Check sheet for the modelled part. Datum: model origin and axes. Units: mm. A direction names the side the tool comes from. Round coordinates to 2 decimals unless told otherwise and drop trailing zeros. Order: outer loops, then holes, each group sorted by start corner. A loop starts at its lowest first (then second) coordinate and runs counter-clockwise, first axis right, second up. Notation, with made-up numbers: M 67,79 L 108,79 A31 ccw 108,112 Z; hole C 18,32.5 d5. An arc over 180 degrees is marked long. One line per item, written item: value. Start each with the question number.
(1) Cross-section at C-C, the plane z = -9.25. Enter the section's corners in (x, y), and give its area (3 significant figures).
(2) Release check for a two-part mould opening along Y. For faces 1 (the face through (4.52, 14.77, -8.5)), 2 (the face through (15.86, 11.62, -1.48)), 3 (the face through (10, 8, 0)), 4 (the face through (13, 0, -10)) record: released by +Y, released by -Y, zero draft, split by the parting line, or undercut.
(3) Access from +Z, -Z, +X, -X, +Y, -Y to the whole of each face (thin tool, end or side, straight path). Record for faces 5 (the face through (3, 12, -12)), 6 (the face through (12, 8, -3)), 7 (the face through (10, 8, -20)).
(4) Thickness scan on L1, parallel to Z at x = 5.25, y = 10; L2, parallel to Y at x = 4.05, z = -10; L3, parallel to Z at x = 12.75, y = 6. Record the ranges inside material, lowest first.
(5) Cross-section at B-B, the plane x = 16. Enter the section's corners in (y, z), and give its area (3 significant figures).
(6) Depth check by flat-ended pin: pin 1 Ø4 at (y, z) = (17, -7) entering from -X; pin 2 Ø6 at (x, z) = (21.5, -11) entering from +Y; pin 3 Ø8 at (y, z) = (9.5, -11) entering from +X. Enter the tip coordinate at first touch or a pass-through.
(7) Cross-section at A-A, the plane y = 2.5. Enter the section's corners in (x, z), and give its area (3 significant figures).
(8) Cross-section at D-D, the plane y = 10.75. Enter the section's corners in (x, z).
from build123d import *

# Parameters (mm, degrees)
SKETCH_1_W          = 40
SKETCH_1_H          = 20
EXTRUDE_1_DEPTH     = 20
SKETCH_2_W          = 34
SKETCH_2_H          = 14
CUT_EXTRUDE_1_DEPTH = 20
CUT_EXTRUDE_2_DEPTH = 20
SKETCH_5_R          = 5
CUT_EXTRUDE_3_DEPTH = 3
SKETCH_6_W          = 34
SKETCH_6_H          = 20
CUT_EXTRUDE_4_DEPTH = 3
SKETCH_7_W          = 14
SKETCH_7_H          = 20
CUT_EXTRUDE_5_DEPTH = 3
EXTRUDE_2_DEPTH     = 3
EXTRUDE_3_DEPTH     = 3


with BuildPart() as part:
    # 草图1 → 凸台-拉伸1 (new body)
    with BuildSketch(Plane(origin=(0, 0, 0), x_dir=(1, 0, 0), z_dir=(0, 1, 0))):
        with Locations((20, 10)):
            Rectangle(SKETCH_1_W, SKETCH_1_H)
    extrude(amount=EXTRUDE_1_DEPTH)

    # 草图2 → 切除-拉伸1 (cut)
    with BuildSketch(Plane.XY):
        with Locations((23, 13)):
            Rectangle(SKETCH_2_W, SKETCH_2_H)
    extrude(amount=-CUT_EXTRUDE_1_DEPTH, mode=Mode.SUBTRACT)

    # 草图4 → 切除-拉伸2 (cut)
    with BuildSketch(Plane.ZY):
        with BuildLine():
            ThreePointArc((-7.4, 10), (-9.005023076, 12.402086785), (-11.838477631, 11.838477631))
            Line((-11.838477631, 11.838477631), (-8.161522369, 8.161522369))
            ThreePointArc((-8.161522369, 8.161522369), (-7.597913215, 9.005023076), (-7.4, 10))
        make_face()
        with BuildLine():
            Line((-8.161522369, 8.161522369), (-11.838477631, 11.838477631))
            ThreePointArc((-11.838477631, 11.838477631), (-11.838477631, 8.161522369), (-8.161522369, 8.161522369))
        make_face()
    extrude(amount=-CUT_EXTRUDE_2_DEPTH, mode=Mode.SUBTRACT)

    # 草图5 → 切除-拉伸3 (cut)
    with BuildSketch(Plane(origin=(6, 0, 0), x_dir=(0, 0, -1), z_dir=(1, 0, 0))):
        with Locations(Location((10, 10, 0), (0, 0, 90))):
            Circle(SKETCH_5_R)
    extrude(amount=-CUT_EXTRUDE_3_DEPTH, mode=Mode.SUBTRACT)

    # 草图6 → 切除-拉伸4 (cut)
    with BuildSketch(Plane(origin=(0, 6, 0), x_dir=(1, 0, 0), z_dir=(0, 1, 0))):
        with Locations((23, 10)):
            Rectangle(SKETCH_6_W, SKETCH_6_H)
    extrude(amount=-CUT_EXTRUDE_4_DEPTH, mode=Mode.SUBTRACT)

    # 草图7 → 切除-拉伸5 (cut)
    with BuildSketch(Plane(origin=(0, 3, 0), x_dir=(1, 0, 0), z_dir=(0, 1, 0))):
        with Locations((33, 10)):
            Rectangle(SKETCH_7_W, SKETCH_7_H)
        with BuildLine():
            ThreePointArc((18.6, 10), (16.994976924, 12.402086785), (14.161522369, 11.838477631))
            Line((14.161522369, 11.838477631), (17.838477631, 8.161522369))
            ThreePointArc((17.838477631, 8.161522369), (18.402086785, 9.005023076), (18.6, 10))
        make_face()
        with BuildLine():
            Line((17.838477631, 8.161522369), (14.161522369, 11.838477631))
            ThreePointArc((14.161522369, 11.838477631), (14.161522369, 8.161522369), (17.838477631, 8.161522369))
        make_face()
    extrude(amount=-CUT_EXTRUDE_5_DEPTH, mode=Mode.SUBTRACT)

    # 草图9 → 凸台-拉伸2 (add)
    with BuildSketch(Plane.XY):
        Polygon((6, 20), (26, 3), (6, 3), align=None)
    extrude(amount=-EXTRUDE_2_DEPTH)

    # 草图10 → 凸台-拉伸3 (add)
    with BuildSketch(Plane(origin=(0, 0, -20), x_dir=(-1, 0, 0), z_dir=(0, 0, -1))):
        Polygon((-26, 3), (-6, 3), (-6, 20), align=None)
    extrude(amount=-EXTRUDE_3_DEPTH)


solid = part.part
Values found:
1. outline: M 0,0 L 13.51,0 L 13.51,3 L 6,3 L 6,5.06 L 3,5.06 L 3,7.51 L 0,7.51 Z; M 0,12.49 L 3,12.49 L 3,14.94 L 6,14.94 L 6,20 L 0,20 Z; M 18.49,0 L 26,0 L 26,3 L 18.49,3 Z
1. area: 120 mm^2
2. face 1: undercut
2. face 2: released by +Y
2. face 3: zero draft
2. face 4: released by -Y
3. face 5: +X
3. face 6: +X, +Y
3. face 7: -Z, +X, -X, +Y, -Y
4. L1: -20 to -15, -5 to 0
4. L2: 0 to 5, 15 to 20
4. L3: -20 to -17, -3 to 0
5. outline: M 0,-20 L 11.5,-20 L 11.5,-17 L 3,-17 L 3,-12.6 L 0,-12.6 Z; M 0,-7.4 L 3,-7.4 L 3,-3 L 11.5,-3 L 11.5,0 L 0,0 Z
5. area: 95.4 mm^2
6. pin 1: x = 0
6. pin 2: y = 3
6. pin 3: x = 6
7. outline: M 0,-20 L 26,-20 L 26,0 L 0,0 Z; hole C 16,-10 d5.2
7. area: 499 mm^2
8. outline: M 0,-20 L 16.88,-20 L 16.88,-17 L 6,-17 L 6,-14.94 L 3,-14.94 L 3,-12.49 L 0,-12.49 Z; M 0,-7.51 L 3,-7.51 L 3,-5.06 L 6,-5.06 L 6,-3 L 16.88,-3 L 16.88,0 L 0,0 Z
